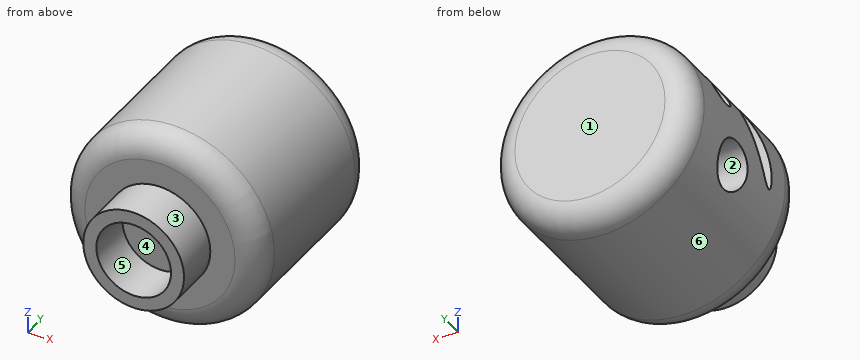
from build123d import *

# Parameters (mm, degrees)
F0_R      = 20.498108569
F1_DEPTH  = 38.354
F2_R      = 5.08
F3_R      = 10.3545358817
F4_DEPTH  = 9.144
F5_R      = 7.6794076655
F4_FACE_R = 10.3545358817
F6_DEPTH  = 20.066
F7_R      = 2.4445782071
F7_R_2    = 4.7073560898
F8_DEPTH  = 51.308


with BuildPart() as f1:
    # F0 (on Front) → F1 (new body)
    with BuildSketch(Plane.XZ):
        Circle(F0_R)
    extrude(amount=-F1_DEPTH)

    # F2
    f2_edges = [f1.edges().sort_by_distance(p)[0] for p in [
        (-20.498109, 0, 0),
        (-20.498109, 38.354, 0),
    ]]
    fillet(f2_edges, radius=F2_R)

    # F3 (on Front) → F4 (join)
    with BuildSketch(Plane.XZ):
        Circle(F3_R)
    extrude(amount=F4_DEPTH)

    # F5 (on Front) + F4_face (on face) → F6 (cut)
    with BuildSketch(Plane.XZ):
        Circle(F5_R)
    with BuildSketch(Plane.XZ.offset(9.144)):
        Circle(F4_FACE_R)
    extrude(amount=F6_DEPTH, mode=Mode.SUBTRACT)

    # F7 (on Right) → F8 (cut)
    with BuildSketch(Plane.YZ):
        with Locations((23.5781669617, 9.1338856146)):
            Circle(F7_R)
        with Locations((22.0204498619, -5.4520084523)):
            Circle(F7_R_2)
        with BuildLine():
            add(Edge.make_bspline(
                [(14.2318671569, 10.691601783), (11.6649759051, 8.7850122349), (5.8643220815, -13.5165030483), (18.8512904338, 7.7362532922), (15.4725782315, 11.6131549519), (14.2318671569, 10.691601783)],
                knots=[0, 0, 0, 0, 0.4118458542, 0.8009336344, 1, 1, 1, 1], degree=3))
        make_face()
    extrude(amount=-F8_DEPTH, mode=Mode.SUBTRACT)


solid = f1.part
Design review of the part built by this model. Coordinates are the model's own, in mm. Face numbers are marked on the shaded views. A direction names the side the tool comes from. Coordinates: 2 decimals unless noted, no trailing zeros. Order: outer loops, then holes, each group sorted by start corner. A loop starts at its lowest first (then second) coordinate and runs counter-clockwise, first axis right, second up. Notation, with made-up numbers: (-6, 17.5) -> (50, 17.5) arc R26 cw to (50, 33.5) -> close; hole circle Ø3 at (62, 46.25). An arc over 180 degrees is marked (long way). Use one line per item in the form item = value. Start each with the question number.
(1) Add section B-B on y = -5. State the section outline as (x, z) points, plus the area to 3 significant figures.
(2) For the marked faces 5 and 6, list the 3-axis set-ups (+Z, -Z, +X, -X, +Y, -Y) from which the entire face can be reached by the end or side of a thin tool; tool diameter is ignored.
(3) Add section D-D on y = 1.5. State the section outline as (x, z) points.
(4) Insertion check: pin 1 (12.5 mm diameter, centred on x = 0, z = 0, fed in from -Y); pin 2 (2 mm diameter, centred on x = -1.5, y = 13.5, fed in from -Z); pin 3 (5.5 mm diameter, centred on y = 24.5, z = 8.5, fed in from -X). Each pin has a flat end and moves straight along its axis. Give the tip position at first contact, or say it passes through.
(5) Add section A-A on y = 22. State the section outline as (x, z) points, plus the area to 3 significant figures.
(6) Add section C-C on x = -13.5. Give the number of separate pieces and of enclosed holes in the cut face, plus the area to 3 significant figures.
(7) The part is to be moulded in two halves that separate along Z. For the marked faces 1, 2, 3 and 4, say which applies: +Z half, -Z half, draft (parallel to the pull), parting line (faces both ways), or undercut.
(8) For probe 1 along Z at (x, y) = (0, -3); probe 2 along Z at (x, y) = (-0.5, 23); probe 3 along Y at (x, z) = (-8, 10.5), list the stretches that pass through material, from the lowest coordinate up.
Answer block:
q1.outline = circle Ø20.71 at (0, 0); hole circle Ø15.36 at (0, 0)
q1.area = 152 mm²
q2.face_5 = -Y
q2.face_6 = +Y, -Y
q3.outline = circle Ø38.04 at (0, 0)
q4.pin_1 = 0
q4.pin_2 = -20.49
q4.pin_3 = -19.68
q5.outline = (-20.48, -0.74) -> (0, -0.74) -> (0, -10.16) -> (-17.8, -10.16) arc R20.5 ccw (long way) to (-17.3, 11) -> (0, 11) -> (0, 7.27) -> (-19.17, 7.27) arc R20.5 ccw to start
q5.area = 1,070 mm²
q6.separate_pieces = 1
q6.enclosed_holes = 3
q6.area = 1,010 mm²
q7.face_1 = draft
q7.face_2 = undercut
q7.face_3 = parting line
q7.face_4 = undercut
q8.probe_1 = -10.35 to -7.68, 7.68 to 10.35
q8.probe_2 = -20.49 to -10.06, -0.85 to 6.76, 11.51 to 20.49
q8.probe_3 = 0 to 14.01, 15.92 to 21.55, 25.61 to 38.35
